```python
from build123d import *

# Parameters (mm, degrees)
F2_W     = 279.4
F2_H     = 50.8
F3_DEPTH = 31.751


with BuildPart() as f1:
    # F0 (on Right) → F1 (revolve)
    with BuildSketch(Plane.YZ):
        Polygon((0, 152.4), (0, 0), (31.75, 0), (31.75, 146.05), (6.35, 146.05), (6.35, 152.4), align=None)
    revolve(axis=Axis((0, 59.051867, 0), (0, 1, 0)))

    # F2 (on face) → F3 (cut, through all)
    with BuildSketch(Plane.XZ):
        Rectangle(F2_W, F2_H)
    extrude(amount=-F3_DEPTH, mode=Mode.SUBTRACT)


solid = f1.part
```
Source: CAD feature listing. Evaluate the final solid. Frame: model axes, mm. A direction names the side the tool comes from. Coordinates: 2 decimals unless noted, no trailing zeros. Loops run counter-clockwise (first coordinate to the right, second up) from the corner with the lowest first, then second, coordinate; pieces in that order, holes last. Notation, with made-up numbers: (30, 42.5) - (65, 42.5) arc R13 ccw to (65, 49.5) - close; hole circle Ø8 at (85, 50). An arc over 180 degrees is marked (long way). Answer as CSV lines item,"result".
1. Section A-A (y = 23). Return loops of the section in (x, z).
Established:
outline,"circle Ø292.1 at (0, 0); hole (-139.7, -25.4) - (139.7, -25.4) - (139.7, 25.4) - (-139.7, 25.4) - close"
2. Contact query for flat-ended pins moving along their axis: pin 1 (6 mm diameter, centred on x = -79, y = 11, fed in from +Z); pin 2 (10 mm diameter, centred on y = 28, z = -92, fed in from +X); pin 3 (4 mm diameter, centred on x = -65.5, y = 23.5, fed in from -Z). Output: stop coordinate, or through.
Established:
pin 1,"stops at z = 124.72"
pin 2,"stops at x = 117.31"
pin 3,"stops at z = -131.52"
3. Ray query, line 1 (Z direction, x = -29, y = 5); line 2 (Z direction, x = -105, y = 3); line 3 (X direction, y = 8, z = -11). Return the intervals inside material, ascending.
Established:
line 1,"z = -149.62 to -25.4, 25.4 to 149.62"
line 2,"z = -110.46 to -25.4, 25.4 to 110.46"
line 3,"x = -145.64 to -139.7, 139.7 to 145.64"
4. Section D-D (z = 108). Return loops of the section in (x, y).
Established:
outline,"(-107.53, 0) - (107.53, 0) - (107.53, 6.35) - (98.32, 6.35) - (98.32, 31.75) - (-98.32, 31.75) - (-98.32, 6.35) - (-107.53, 6.35) - close"
5. Reachability of faces 4 (the flat face through (139.7, 16, 0)), 5 (the cylindrical face through (43.869, 18.872, 139.306)), 6 (the flat face through (2, 31.75, -30)) from +Z, -Z, +X, -X, +Y, -Y: full face, straight path, thin tool, end or side. Return the list, or none.
Established:
face 4,"+Y, -Y"
face 5,"+Y"
face 6,"+Z, -Z, +X, -X, +Y"
6. Mould query, pull axis Z, two halves, no side actions, for faces 1 (the flat face through (2, 0, 32)), 2 (the flat face through (-2, 16, -25.4)), 3 (the cylindrical face through (-92.73, 3.13, -120.94)). Classes: released by +Z, released by -Z, zero draft, split by the parting line, or undercut.
Established:
face 1,"zero draft"
face 2,"undercut"
face 3,"split by the parting line"
7. Section C-C (z = 0). Return loops of the section in (x, y), then the cut area to 3 significant figures.
Established:
outline,"(-152.4, 0) - (-139.7, 0) - (-139.7, 31.75) - (-146.05, 31.75) - (-146.05, 6.35) - (-152.4, 6.35) - close; (139.7, 0) - (152.4, 0) - (152.4, 6.35) - (146.05, 6.35) - (146.05, 31.75) - (139.7, 31.75) - close"
area,"484 mm2"
8. Section B-B (x = 0). Return loops of the section in (y, z).
Established:
outline,"(0, -152.4) - (6.35, -152.4) - (6.35, -146.05) - (31.75, -146.05) - (31.75, -25.4) - (0, -25.4) - close; (0, 25.4) - (31.75, 25.4) - (31.75, 146.05) - (6.35, 146.05) - (6.35, 152.4) - (0, 152.4) - close"
